from build123d import *

# Parameters (mm, degrees)
SKETCH1_R           = 4.5
BOSS_EXTRUDE1_DEPTH = 1.5748
SKETCH2_W           = 5
SKETCH2_H           = 5
BOSS_EXTRUDE2_DEPTH = 1
SKETCH3_W           = 3.5
SKETCH3_H           = 4
BOSS_EXTRUDE3_DEPTH = 0.1


with BuildPart() as part:
    # Sketch1 → Boss-Extrude1 (new body)
    with BuildSketch(Plane(origin=(0, 0, 0), x_dir=(1, 0, 0), z_dir=(0, 1, 0))):
        Circle(SKETCH1_R)
    extrude(amount=BOSS_EXTRUDE1_DEPTH)

    # Sketch2 → Boss-Extrude2 (add)
    with BuildSketch(Plane(origin=(0, 1.5748, 0), x_dir=(1, 0, 0), z_dir=(0, 1, 0))):
        Rectangle(SKETCH2_W, SKETCH2_H)
    extrude(amount=BOSS_EXTRUDE2_DEPTH)

    # Sketch3 → Boss-Extrude3 (add)
    with BuildSketch(Plane(origin=(0, 2.5748, 0), x_dir=(1, 0, 0), z_dir=(0, 1, 0))):
        with Locations((0.25, 0)):
            Rectangle(SKETCH3_W, SKETCH3_H)
    extrude(amount=BOSS_EXTRUDE3_DEPTH)


solid = part.part
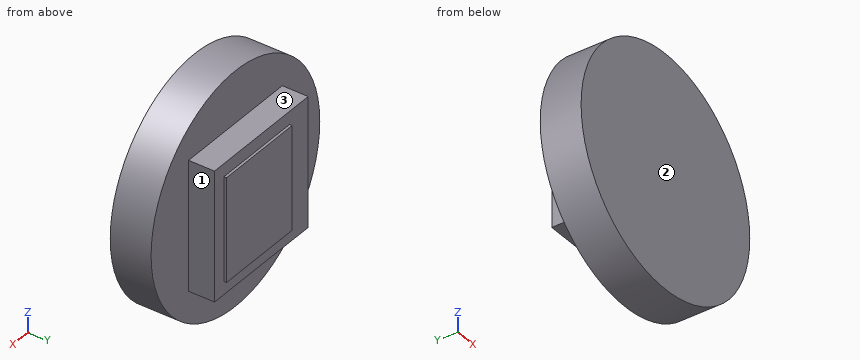
Read the model definition and answer for the solid it produces. Units are mm, in the model's axes. Face numbers are marked on the shaded views. A direction names the side the tool comes from. Give positions to 0.01 mm unless a question says otherwise; leave off trailing zeros. Write each loop counter-clockwise with the first axis right and the second up, starting at its lowest first coordinate (ties: lowest second). Pieces come first, ordered by that corner, then holes. Notation, with made-up numbers: (2.5, 67.25) - (40.5, 67.25) arc R16 ccw to (40.5, 92.25) - close; hole circle Ø5 at (53, 21.5). An arc over 180 degrees is marked (long way). Return JSON: item names as keys, results as strings.
Q1. Consider line 1 along Y through (x, z) = (3.75, -1.5); line 2 along X through (y, z) = (2.45, -0.5). Determine where each line is inside the solid, lowest interval first. Write a range as [from, to].
Reply:
{"line 1": "[0, 1.57]", "line 2": "[-2.5, 2.5]"}
Q2. A cutting plane is placed at B-B, the plane z = 0. Determine the outline of the cut face in (x, y), and give its area (3 significant figures).
Reply:
{"outline": "(-4.5, 0) - (4.5, 0) - (4.5, 1.57) - (2.5, 1.57) - (2.5, 2.57) - (2, 2.57) - (2, 2.67) - (-1.5, 2.67) - (-1.5, 2.57) - (-2.5, 2.57) - (-2.5, 1.57) - (-4.5, 1.57) - close", "area": "19.5 mm²"}
Q3. A cutting plane is placed at A-A, the plane x = 0. Determine the outline of the cut face in (y, z).
Reply:
{"outline": "(0, -4.5) - (1.57, -4.5) - (1.57, -2.5) - (2.57, -2.5) - (2.57, -2) - (2.67, -2) - (2.67, 2) - (2.57, 2) - (2.57, 2.5) - (1.57, 2.5) - (1.57, 4.5) - (0, 4.5) - close"}
Q4. A cutting plane is placed at C-C, the plane y = 2.1. Determine the outline of the cut face in (x, z), and give its area (3 significant figures).
Reply:
{"outline": "(-2.5, -2.5) - (2.5, -2.5) - (2.5, 2.5) - (-2.5, 2.5) - close", "area": "25.0 mm²"}
Q5. A cutting plane is placed at D-D, the plane y = 1.1. Determine the outline of the cut face in (x, z).
Reply:
{"outline": "circle Ø9 at (0, 0)"}
Q6. Given P1, Ø0.5, axis at y = 2, z = -0.5, coming from the +X side; P2, Ø1.1, axis at x = 0.5, y = 2.5, coming from the +Z side; P3, Ø0.5, axis at y = 2, z = 1, coming from the -X side, each flat-ended and moving along its own axis, determine where each tip first touches the part or whether it passes through.
Reply:
{"P1": "x = 2.5", "P2": "z = 2.5", "P3": "x = -2.5"}
Q7. For the marked faces 1, 2 and 3, determine the directions among +Z, -Z, +X, -X, +Y, -Y from which every point of the face is accessible in a straight line to the end or side of a thin tool.
Reply:
{"face 1": "+Z, -Z, +X, +Y", "face 2": "+Z, -Z, +X, -X, -Y", "face 3": "+Z, +X, -X, +Y"}
